```python
from build123d import *

# Parameters (mm, degrees)
BOSS_EXTRUDE1_DEPTH      = 2
BOSS_EXTRUDE2_DEPTH      = 8
SKETCH24_R               = 3.9
BOSS_EXTRUDE5_DEPTH      = 4.4
SKETCH30_W               = 4.40861202
SKETCH30_H               = 1.324178481
CUT_EXTRUDE12_DEPTH      = 16
CUT_EXTRUDE11_DEPTH      = 23.928148639
FILLET1_R                = 1.5
SKETCH34_R               = 0.75
CUT_EXTRUDE13_DEPTH      = 8
SKETCH35_R               = 0.75
CUT_EXTRUDE14_DEPTH      = 3
CUT_EXTRUDE14_DEPTH_BACK = 8
SKETCH36_R               = 0.95
CUT_EXTRUDE15_DEPTH      = 8
SKETCH37_R               = 2
CUT_EXTRUDE16_DEPTH      = 4.5
SKETCH38_W               = 3
SKETCH38_H               = 1.25
CUT_EXTRUDE17_DEPTH      = 3.6


with BuildPart() as part:
    # Sketch2 → Boss-Extrude1 (new body)
    with BuildSketch(Plane.XY):
        with BuildLine():
            Line((-2.5, 7.5), (-16.7, 7.5))
            Line((-16.7, 7.5), (-20.7, 3.793442666))
            Line((-20.7, 3.793442666), (-20.7, -4.031648778))
            Line((-20.7, -4.031648778), (-15.7, -7.5))
            Line((-15.7, -7.5), (-6.7, -7.5))
            Line((-6.7, -7.5), (-4.2, -5.6))
            ThreePointArc((-4.2, -5.6), (3.130495168, -6.260990337), (7, 0))
            ThreePointArc((7, 0), (4.949747468, 4.949747468), (0, 7))
            Line((0, 7), (0, 7.5))
            Line((0, 7.5), (-2.5, 7.5))
        make_face()
    extrude(amount=BOSS_EXTRUDE1_DEPTH)

    # Sketch4 → Boss-Extrude2 (add)
    with BuildSketch(Plane.XY.offset(2)):
        Polygon((-15.7, -7.5), (-6.7, -7.5), (-6.759079174, -4.5), (-7.7, -4.5), (-7.7, 2), (-5.5, 2), (-5.5, 5.3), (-2.5, 5.3), (-2.5, 7.5), (-16.7, 7.5), (-20.7, 3.793442666), (-20.7, -4.031648778), align=None)
    extrude(amount=BOSS_EXTRUDE2_DEPTH)

    # Sketch24 → Boss-Extrude5 (add)
    with BuildSketch(Plane.XY.offset(2)):
        Circle(SKETCH24_R)
    extrude(amount=BOSS_EXTRUDE5_DEPTH)

    # Sketch30 → Cut-Extrude12 (cut)
    with BuildSketch(Plane(origin=(-5.5, 0, 0), x_dir=(0, 0, -1), z_dir=(1, 0, 0))):
        with Locations((-4.20430601, 4.63791076)):
            Rectangle(SKETCH30_W, SKETCH30_H)
    extrude(amount=-CUT_EXTRUDE12_DEPTH, mode=Mode.SUBTRACT)

    # Sketch28 → Cut-Extrude11 (cut, through all)
    with BuildSketch(Plane.XY.offset(6.4)):
        with BuildLine():
            Line((-1, 1.732050808), (-1, -1.732050808))
            ThreePointArc((-1, -1.732050808), (2, 0), (-1, 1.732050808))
        make_face()
    extrude(amount=-CUT_EXTRUDE11_DEPTH, mode=Mode.SUBTRACT)

    # Fillet1
    # the kernel refuses this fillet: 1.5 mm, written as the material it takes off along each edge
    with BuildSketch(Plane(origin=(-15.230677435, -6, 1.5), x_dir=(-0.5699665637840448, -0.8216678867816415, 0), z_dir=(0, 0, -1))) as fillet1_piece_1_section:
        Polygon((0, 0), (FILLET1_R * 1.02, 0), (FILLET1_R * 1.02, -FILLET1_R * 0.319139344377), (FILLET1_R * 0.838101244517, -FILLET1_R * 0.58136589506), align=None)
    fillet1_piece_1 = extrude(amount=FILLET1_R * 1.02, mode=Mode.PRIVATE)
    fillet1_piece_1 = fillet1_piece_1 - Plane(origin=(-15.230677435, -6, 1.5), x_dir=(0.29860685961507855, 0.9543762064253388, 0), z_dir=(0, 0, -1)) * Sphere(FILLET1_R, mode=Mode.PRIVATE)
    add(fillet1_piece_1, mode=Mode.SUBTRACT)
    with BuildSketch(Plane(origin=(-16.11186344, 6, 1.5), x_dir=(-0.6796897201843015, 0.7334997506991983, 0), z_dir=(0, 0, -1))) as fillet1_piece_2_section:
        Polygon((0, 0), (FILLET1_R * 1.02, 0), (FILLET1_R * 1.02, FILLET1_R * 0.399932860855), (FILLET1_R * 0.748169745713, FILLET1_R * 0.693283514588), align=None)
    fillet1_piece_2 = extrude(amount=FILLET1_R * 1.02, mode=Mode.PRIVATE)
    fillet1_piece_2 = fillet1_piece_2 - Plane(origin=(-16.11186344, 6, 1.5), x_dir=(0.3650344157067945, -0.9309940254102596, 0), z_dir=(0, 0, -1)) * Sphere(FILLET1_R, mode=Mode.PRIVATE)
    add(fillet1_piece_2, mode=Mode.SUBTRACT)
    with BuildSketch(Plane(origin=(-19.2, 3.138411196, 1.5), x_dir=(-0.6796897201843015, 0.7334997506991983, 0), z_dir=(0, 0, -1))) as fillet1_piece_3_section:
        Polygon((0, 0), (FILLET1_R * 1.02, 0), (FILLET1_R * 1.02, -FILLET1_R * 0.445421399395), (FILLET1_R * 0.693283514588, -FILLET1_R * 0.748169745713), align=None)
    fillet1_piece_3 = extrude(amount=FILLET1_R * 1.02, mode=Mode.PRIVATE)
    fillet1_piece_3 = fillet1_piece_3 - Plane(origin=(-19.2, 3.138411196, 1.5), x_dir=(0.9164304993244992, -0.40019387789901173, 0), z_dir=(0, 0, -1)) * Sphere(FILLET1_R, mode=Mode.PRIVATE)
    add(fillet1_piece_3, mode=Mode.SUBTRACT)
    with BuildSketch(Plane(origin=(-19.2, -3.246599046, 1.5), x_dir=(-0.5699665637840448, -0.8216678867816415, 0), z_dir=(0, 0, -1))) as fillet1_piece_4_section:
        Polygon((0, 0), (FILLET1_R * 1.02, 0), (FILLET1_R * 1.02, FILLET1_R * 0.533833817771), (FILLET1_R * 0.58136589506, FILLET1_R * 0.838101244517), align=None)
    fillet1_piece_4 = extrude(amount=FILLET1_R * 1.02, mode=Mode.PRIVATE)
    fillet1_piece_4 = fillet1_piece_4 - Plane(origin=(-19.2, -3.246599046, 1.5), x_dir=(0.8859928227090906, 0.46369895202380795, 0), z_dir=(0, 0, -1)) * Sphere(FILLET1_R, mode=Mode.PRIVATE)
    add(fillet1_piece_4, mode=Mode.SUBTRACT)
    with BuildSketch(Plane(origin=(-15.230677435, -7.5, 0), x_dir=(0, 1, 0), z_dir=(1, 0, 0))) as fillet1_piece_5_section:
        with BuildLine():
            CenterArc((FILLET1_R, FILLET1_R), FILLET1_R, 180, 90)
            Line((0, FILLET1_R), (0, 0))
            Line((0, 0), (FILLET1_R, 0))
        make_face()
    fillet1_piece_5 = extrude(amount=12.280677435, mode=Mode.PRIVATE)
    fillet1_piece_5 = split(fillet1_piece_5, bisect_by=Plane(origin=(-9.092127217, -9.318016685, 0.3282266), z_dir=(-0.6050832675335577, 0.7961621941231027, 0)), keep=Keep.TOP, mode=Mode.PRIVATE)
    add(fillet1_piece_5, mode=Mode.SUBTRACT)
    with BuildSketch(Plane(origin=(3.75, 7.5, 0), x_dir=(0, 0, 1), z_dir=(-1, 0, 0))) as fillet1_piece_6:
        with BuildLine():
            CenterArc((FILLET1_R, -FILLET1_R), FILLET1_R, 90, 90)
            Line((0, -FILLET1_R), (0, 0))
            Line((0, 0), (FILLET1_R, 0))
        make_face()
    extrude(amount=19.86186344, mode=Mode.SUBTRACT)
    with BuildSketch(Plane(origin=(-17.13139802, 7.100249626, 0), x_dir=(0.6796897201843014, -0.7334997506991981, 0), z_dir=(-0.7334997506991983, -0.6796897201843015, 0))) as fillet1_piece_7:
        with BuildLine():
            CenterArc((FILLET1_R, FILLET1_R), FILLET1_R, 180, 90)
            Line((0, FILLET1_R), (0, 0))
            Line((0, 0), (FILLET1_R, 0))
        make_face()
    extrude(amount=4.21013989, mode=Mode.SUBTRACT)
    with BuildSketch(Plane(origin=(-20.054949846, -4.479100876, 0), x_dir=(0.5699665637840448, 0.8216678867816416, 0), z_dir=(0.8216678867816415, -0.5699665637840448, 0))) as fillet1_piece_8:
        with BuildLine():
            CenterArc((FILLET1_R, FILLET1_R), FILLET1_R, 180, 90)
            Line((0, FILLET1_R), (0, 0))
            Line((0, 0), (FILLET1_R, 0))
        make_face()
    extrude(amount=4.830811364, mode=Mode.SUBTRACT)
    with BuildSketch(Plane(origin=(-20.7, 3.138411196, 0), x_dir=(1, 0, 0), z_dir=(0, -1, 0))) as fillet1_piece_9:
        with BuildLine():
            CenterArc((FILLET1_R, FILLET1_R), FILLET1_R, 180, 90)
            Line((0, FILLET1_R), (0, 0))
            Line((0, 0), (FILLET1_R, 0))
        make_face()
    extrude(amount=6.385010242, mode=Mode.SUBTRACT)
    with BuildSketch(Plane(origin=(-15.7, -7.5, 1.5), x_dir=(1, 0, 0), z_dir=(0, 0, 1))) as fillet1_piece_10:
        with BuildLine():
            CenterArc((FILLET1_R * 0.312881710173, FILLET1_R), FILLET1_R, 235.252105822, 34.747894178)
            Line((-FILLET1_R * 0.257084853611, FILLET1_R * 0.178332113218), (0, 0))
            Line((0, 0), (FILLET1_R * 0.312881710173, 0))
        make_face()
    extrude(amount=9.673306413, mode=Mode.SUBTRACT)
    with BuildSketch(Plane(origin=(-20.7, -4.031648778, 1.5), x_dir=(0, 1, 0), z_dir=(0, 0, 1))) as fillet1_piece_11:
        with BuildLine():
            CenterArc((FILLET1_R * 0.523366488011, -FILLET1_R), FILLET1_R, 90, 55.252105822)
            Line((-FILLET1_R * 0.298301398771, -FILLET1_R * 0.430033436216), (0, 0))
            Line((0, 0), (FILLET1_R * 0.523366488011, 0))
        make_face()
    extrude(amount=10.46262433, mode=Mode.SUBTRACT)
    with BuildSketch(Plane(origin=(-20.7, 3.793442666, 1.5), x_dir=(0.7334997506991984, 0.6796897201843014, 0), z_dir=(0, 0, 1))) as fillet1_piece_12:
        with BuildLine():
            CenterArc((FILLET1_R * 0.436687646465, -FILLET1_R), FILLET1_R, 90, 47.18059856)
            Line((-FILLET1_R * 0.296812104234, -FILLET1_R * 0.320310279816), (0, 0))
            Line((0, 0), (FILLET1_R * 0.436687646465, 0))
        make_face()
    extrude(amount=10.137578674, mode=Mode.SUBTRACT)
    with BuildSketch(Plane(origin=(-16.7, 7.5, 1.5), x_dir=(1, 0, 0), z_dir=(0, 0, 1))) as fillet1_piece_13:
        with BuildLine():
            CenterArc((FILLET1_R * 0.392091040054, -FILLET1_R), FILLET1_R, 90, 42.81940144)
            Line((-FILLET1_R * 0.287598680131, -FILLET1_R * 0.266500249301), (0, 0))
            Line((0, 0), (FILLET1_R * 0.392091040054, 0))
        make_face()
    extrude(amount=9.9703414, mode=Mode.SUBTRACT)

    # Sketch34 → Cut-Extrude13 (cut, along a direction that is not the sketch's normal)
    with BuildSketch(Plane.XZ.offset(-2)):
        with Locations((-7, 10)):
            Circle(SKETCH34_R)
    extrude(amount=-CUT_EXTRUDE13_DEPTH, dir=(0.6685833876565112, -0.7436371788377336, 0), mode=Mode.SUBTRACT)

    # Sketch35 → Cut-Extrude14 (cut, two sides, along a direction that is not the sketch's normal)
    with BuildSketch(Plane(origin=(0, -4.5, 0), x_dir=(1, 0, 0), z_dir=(0, 1, 0))) as cut_extrude14_sk:
        with Locations((-8.259079174, -10)):
            Circle(SKETCH35_R)
    extrude(amount=CUT_EXTRUDE14_DEPTH, dir=(0.5999194182208608, 0.8000604299935998, 0), mode=Mode.SUBTRACT)
    extrude(cut_extrude14_sk.sketch, amount=-CUT_EXTRUDE14_DEPTH_BACK, dir=(0.5999194182208608, 0.8000604299935998, 0), mode=Mode.SUBTRACT)

    # Sketch36 → Cut-Extrude15 (cut)
    with BuildSketch(Plane.XY.offset(10)):
        with Locations((-11.7, 0)):
            Circle(SKETCH36_R)
        with Locations((-16.7, 0)):
            Circle(SKETCH36_R)
    extrude(amount=-CUT_EXTRUDE15_DEPTH, mode=Mode.SUBTRACT)

    # Sketch37 → Cut-Extrude16 (cut)
    with BuildSketch(Plane(origin=(0, 0, 0), x_dir=(-1, 0, 0), z_dir=(0, 0, -1))):
        with Locations((11.7, 0)):
            Circle(SKETCH37_R)
        with Locations((16.7, 0)):
            Circle(SKETCH37_R)
    extrude(amount=-CUT_EXTRUDE16_DEPTH, mode=Mode.SUBTRACT)

    # Sketch38 → Cut-Extrude17 (cut)
    with BuildSketch(Plane.XY.offset(10)):
        with Locations((-4, 5.925)):
            Rectangle(SKETCH38_W, SKETCH38_H)
    extrude(amount=-CUT_EXTRUDE17_DEPTH, mode=Mode.SUBTRACT)


solid = part.part
```
The listing builds one solid part. Answer for the finished solid, in the listing's coordinates (mm). A direction names the side the tool comes from. Coordinates: 2 decimals unless noted, no trailing zeros. Write each loop counter-clockwise with the first axis right and the second up, starting at its lowest first coordinate (ties: lowest second). Pieces come first, ordered by that corner, then holes. Notation, with made-up numbers: M 74,47 L 95,47 A27 cw 95,85 Z; hole C 47,54 d7. An arc over 180 degrees is marked long. Use a Markdown table: item, result. Add a question column.
1. Straight lines are drawn through the part: line 1 along Y through (x, z) = (-7.25, 5.25); line 2 along Y through (x, z) = (-11.7, 3.25); line 3 along Y through (x, z) = (-8, 3.5). For each, find the intervals that lie inside material, in ascending order. Write a range as [from, to].
2. Given P1, Ø2, axis at x = -16, y = -0.5, coming from the -Z side; P2, Ø0.7, axis at y = 6.5, z = 8, coming from the +X side; P3, Ø1, axis at y = 4, z = 2.5, coming from the -X side, each flat-ended and moving along its own axis, determine where each tip first touches the part or whether it passes through.
3. For a pull along X with two mould halves and no side action, classify faces 4 (the flat face through (-6, 0, 0)), 5 (the flat face through (-18, 0, 4.5)), 6 (the cylindrical face through (-18.36, 5.38, 0.45)) as +X half, -X half, draft (parallel to the pull), parting line (faces both ways), or undercut.
4. Section C-C (x = -0.5) is taken. Give the vertices of the cut face in (y, z), plus the area to 3 significant figures.
5. Section B-B (x = -14) is taken. Give the vertices of the cut face in (y, z).
6. Section A-A (z = 2.5) is taken. Give the vertices of the cut face in (x, y), plus the area to 3 significant figures.
7. Which of the six approach directions +Z, -Z, +X, -X, +Y, -Y give full straight-line access (tool end or side, diameter ignored) to faces 1 (the flat face through (-4, 6.55, 8)), 2 (the cylindrical face through (-12.623, -1.774, 2.218)), 3 (the flat face through (-7, -4.5, 6))?
Data:
| question | item | result |
|---|---|---|
| 1 | line 1 | y = [-7.5, -4.5], [2, 3.98], [5.3, 7.5] |
| 1 | line 2 | y = [-7.5, -2], [2, 3.98], [5.3, 7.5] |
| 1 | line 3 | y = [-7.5, 3.98], [5.3, 7.5] |
| 2 | P1 | stops at z = 4.5 |
| 2 | P2 | stops at x = -2.5 |
| 2 | P3 | stops at x = -20.66 |
| 3 | face 4 | draft |
| 3 | face 5 | undercut |
| 3 | face 6 | -X half |
| 4 | outline | M -6.98,0 L -1.94,0 L -1.94,6.4 L -3.87,6.4 L -3.87,2 L -6.98,2 Z; M 1.94,0 L 6,0 A1.5 ccw 7.5,1.5 L 7.5,2 L 3.87,2 L 3.87,6.4 L 1.94,6.4 Z |
| 4 | area | 37.7 mm2 |
| 5 | outline | M -7.5,1.5 A1.5 ccw -6,0 L 6,0 A1.5 ccw 7.5,1.5 L 7.5,10 L -7.5,10 Z; hole M 3.98,2 L 5.3,2 L 5.3,6.41 L 3.98,6.41 Z |
| 6 | outline | M -20.7,-3.25 A1.5 ccw -20.05,-4.48 L -16.09,-7.23 A1.5 ccw -15.23,-7.5 L -6.7,-7.5 L -6.76,-4.5 L -7.7,-4.5 L -7.7,2 L -5.5,2 L -5.5,3.98 L -20.44,3.98 A1.5 ccw -20.7,3.14 Z; M -19.07,5.3 L -2.5,5.3 L -2.5,7.5 L -16.11,7.5 A1.5 ccw -17.13,7.1 Z; C 0,0 d7.8; hole C -16.7,0 d4; hole C -11.7,0 d4; hole M -1,-1.73 A2 ccw long -1,1.73 Z |
| 6 | area | 194 mm2 |
| 7 | face 1 | +Z, +X, -Y |
| 7 | face 2 | -Z |
| 7 | face 3 | +Z, +X |
